For this review, use the dimensioned drawing (mm, ordinates from the lowest corner) and the shaded views. Round coordinates to 2 decimals unless told otherwise and drop trailing zeros. Write each loop counter-clockwise with the first axis right and the second up, starting at its lowest first coordinate (ties: lowest second). Pieces come first, ordered by that corner, then holes. Notation, with made-up numbers: M 26.5,43.25 L 51.5,43.25 A25 ccw 51.5,58.25 Z; hole C -22.5,46 d2. An arc over 180 degrees is marked long. One line per question, with ' | ' between items.
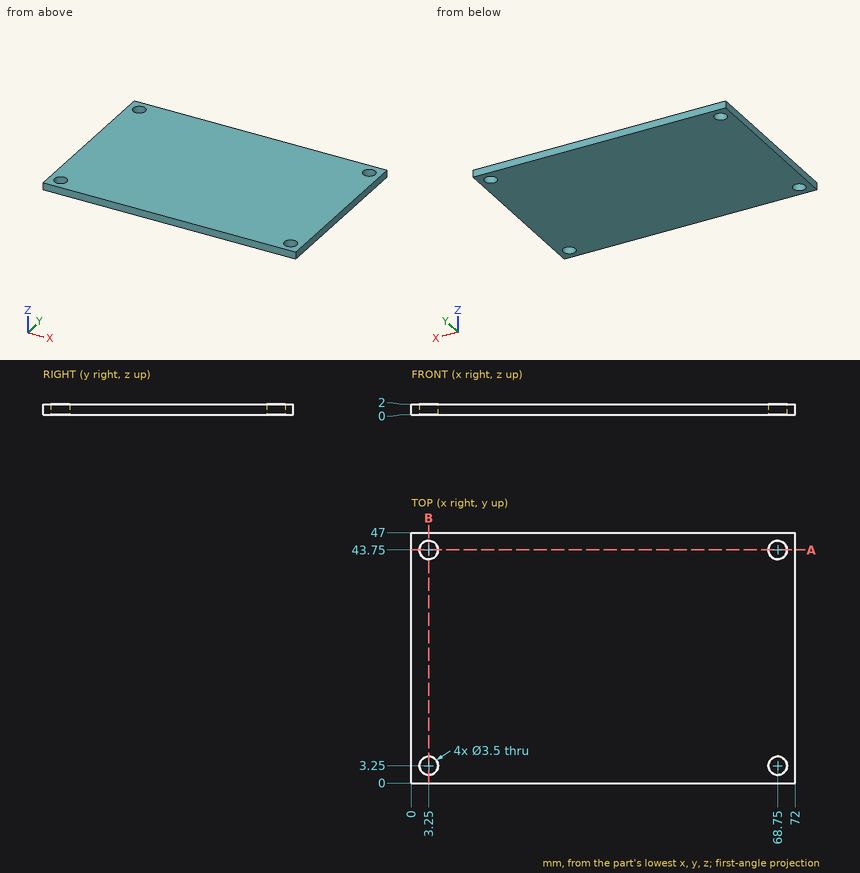
Item 1: Take a section at A-A (y = 43.75). Write out the cut boundary in (x, z), then the cut area to 3 significant figures.
Results:
outline: M 0,0 L 1.5,0 L 1.5,2 L 0,2 Z; M 5,0 L 67,0 L 67,2 L 5,2 Z; M 70.5,0 L 72,0 L 72,2 L 70.5,2 Z | area: 130 mm2
Item 2: Take a section at B-B (x = 3.25). Write out the cut boundary in (y, z), then the cut area to 3 significant figures.
Results:
outline: M 0,0 L 1.5,0 L 1.5,2 L 0,2 Z; M 5,0 L 42,0 L 42,2 L 5,2 Z; M 45.5,0 L 47,0 L 47,2 L 45.5,2 Z | area: 80.0 mm2
Item 3: To check wall thickness, follow line 1 along X through (y, z) = (43.75, 1.05); line 2 along Y through (x, z) = (68.75, 0.65); line 3 along Y through (x, z) = (69.5, 0.9). State the ranges of each line that lie inside material, in increasing order. Write a range as from..to.
Results:
line 1: 0..1.5, 5..67, 70.5..72 | line 2: 0..1.5, 5..42, 45.5..47 | line 3: 0..1.67, 4.83..42.17, 45.33..47
Item 4: Insertion check: pin 1 Ø1.5 at (x, y) = (26, 23.5) entering from -Z. The pin has a flat end and moves straight along its axis. Give the tip position at first contact, or say it passes through.
Results:
pin 1: z = 0
